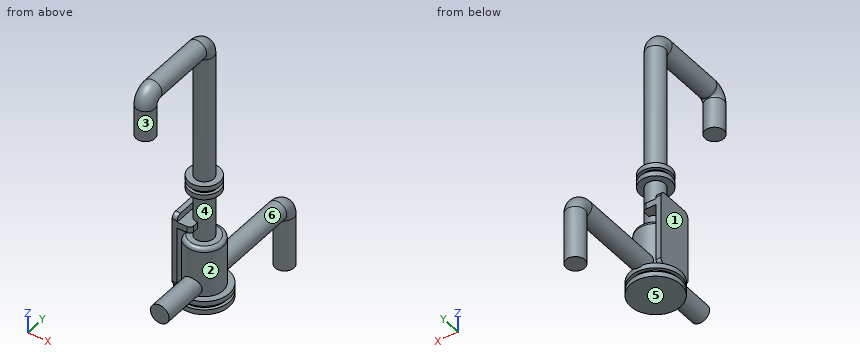
```python
from build123d import *

# Parameters (mm, degrees)
F1_R      = 0.75
F3_R      = 1.5
F3_R_2    = 0.75
F4_DEPTH  = 4
F6_DEPTH  = 6
F7_R      = 0.4
F8_R      = 2
F9_DEPTH  = 0.4
F10_R     = 1.75
F11_DEPTH = 0.3
F12_R     = 2
F12_R_2   = 1.75
F13_DEPTH = 0.4
F14_W     = 3
F14_H     = 0.5
F15_DEPTH = 1.5
F16_R     = 0.3
F18_R     = 1.25
F18_R_2   = 0.75
F19_DEPTH = 0.4
F20_R     = 1
F20_R_2   = 0.75
F21_DEPTH = 0.3
F22_R     = 1.25
F22_R_2   = 1
F22_R_3   = 0.75
F23_DEPTH = 0.4
F24_R     = 0.3
F27_R     = 0.75


with BuildPart() as f2:
    # F2: sweep along a path in F0
    with BuildLine(Plane.YZ) as f2_path:
        Line((0, 0), (0, 2.5))
        ThreePointArc((0, 2.5), (0.2343145751, 3.0656854249), (0.8, 3.3))
        Line((0.8, 3.3), (5.8, 3.3))
        ThreePointArc((5.8, 3.3), (6.3656854249, 3.0656854249), (6.6, 2.5))
        Line((6.6, 2.5), (6.6, -16.7))
    # F1 (on Top) → F2 (sweep)
    with BuildSketch(Plane.XY):
        Circle(F1_R)
    sweep(path=f2_path.line)

    # F3 (on face) → F4 (join)
    with BuildSketch(Plane(origin=(0, 0, -16.7), x_dir=(1, 0, 0), z_dir=(0, 0, -1))):
        with Locations((0, -6.6)):
            Circle(F3_R)
        with Locations((0, -6.6)):
            Circle(F3_R_2, mode=Mode.SUBTRACT)
    extrude(amount=-F4_DEPTH)

    # F5 (on face) → F6 (join)
    with BuildSketch(Plane(origin=(0, 0, -16.7), x_dir=(1, 0, 0), z_dir=(0, 0, -1))):
        with BuildLine():
            ThreePointArc((-1.1, -7.6198039027), (-1.3964240044, -7.1477225575), (-1.5, -6.6))
            Line((-1.5, -6.6), (-1.5, -8.1))
            Line((-1.5, -8.1), (-1.1, -8.1))
            Line((-1.1, -8.1), (-1.1, -7.6198039027))
        make_face()
        with BuildLine():
            Line((-1.5, -5.1), (-1.5, -6.6))
            ThreePointArc((-1.5, -6.6), (-1.3964240044, -6.0522774425), (-1.1, -5.5801960973))
            Line((-1.1, -5.5801960973), (-1.1, -5.1))
            Line((-1.1, -5.1), (-1.5, -5.1))
        make_face()
        with BuildLine():
            ThreePointArc((-1.1, -5.5801960973), (-1.3964240044, -6.0522774425), (-1.5, -6.6))
            ThreePointArc((-1.5, -6.6), (-1.3964240044, -7.1477225575), (-1.1, -7.6198039027))
            Line((-1.1, -7.6198039027), (-1.1, -5.5801960973))
        make_face()
    extrude(amount=-F6_DEPTH)

    # F7
    f7_edges = [f2.edges().sort_by_distance(p)[0] for p in [
        (-1.3, 8.1, -10.7),
        (-1.3, 5.1, -10.7),
        (-1.3, 8.1, -16.7),
        (-1.3, 5.1, -16.7),
    ]]
    fillet(f7_edges, radius=F7_R)

    # F8 (on face) → F9 (join)
    with BuildSketch(Plane(origin=(0, 0, -16.7), x_dir=(1, 0, 0), z_dir=(0, 0, -1))):
        with Locations((0, -6.6)):
            Circle(F8_R)
        with BuildLine():
            Line((-1.1, -5.5), (-1.1, -5.5801960973))
            ThreePointArc((-1.1, -5.5801960973), (1.5, -6.6), (-1.1, -7.6198039027))
            Line((-1.1, -7.6198039027), (-1.1, -7.7))
            Line((-1.1, -7.7), (-1.5, -7.7))
            Line((-1.5, -7.7), (-1.5, -6.6))
            Line((-1.5, -6.6), (-1.5, -5.5))
            Line((-1.5, -5.5), (-1.1, -5.5))
        make_face(mode=Mode.SUBTRACT)
        with BuildLine():
            ThreePointArc((-1.1, -7.6198039027), (1.5, -6.6), (-1.1, -5.5801960973))
            Line((-1.1, -5.5801960973), (-1.1, -5.5))
            Line((-1.1, -5.5), (-1.5, -5.5))
            Line((-1.5, -5.5), (-1.5, -6.6))
            Line((-1.5, -6.6), (-1.5, -7.7))
            Line((-1.5, -7.7), (-1.1, -7.7))
            Line((-1.1, -7.7), (-1.1, -7.6198039027))
        make_face()
    extrude(amount=F9_DEPTH)

    # F10 (on face) → F11 (join)
    with BuildSketch(Plane(origin=(0, 0, -17.1), x_dir=(1, 0, 0), z_dir=(0, 0, -1))):
        with Locations((0, -6.6)):
            Circle(F10_R)
    extrude(amount=F11_DEPTH)

    # F12 (on face) → F13 (join)
    with BuildSketch(Plane(origin=(0, 0, -17.4), x_dir=(1, 0, 0), z_dir=(0, 0, -1))):
        with Locations((0, -6.6)):
            Circle(F12_R)
        with Locations((0, -6.6)):
            Circle(F12_R_2, mode=Mode.SUBTRACT)
        with Locations((0, -6.6)):
            Circle(F12_R_2)
    extrude(amount=F13_DEPTH)

    # F14 (on face) → F15 (join, through all)
    with BuildSketch(Plane(origin=(-1.5, 0, 0), x_dir=(0, -1, 0), z_dir=(-1, 0, 0))):
        with Locations((-6.6, -11.45)):
            Rectangle(F14_W, F14_H)
    extrude(amount=-F15_DEPTH)

    # F16
    f16_edges = [f2.edges().sort_by_distance(p)[0] for p in [
        (0, 8.1, -11.45),
        (0, 5.1, -11.45),
    ]]
    fillet(f16_edges, radius=F16_R)

    # F18 (on offset) → F19 (join)
    with BuildSketch(Plane(origin=(0, 0, -8.8), x_dir=(1, 0, 0), z_dir=(0, 0, -1))):
        with Locations((0, -6.6)):
            Circle(F18_R)
        with Locations((0, -6.6)):
            Circle(F18_R_2, mode=Mode.SUBTRACT)
    extrude(amount=-F19_DEPTH)

    # F20 (on face) → F21 (join)
    with BuildSketch(Plane.XY.offset(-8.4)):
        with Locations((0, 6.6)):
            Circle(F20_R)
        with Locations((0, 6.6)):
            Circle(F20_R_2, mode=Mode.SUBTRACT)
    extrude(amount=F21_DEPTH)

    # F22 (on face) → F23 (join)
    with BuildSketch(Plane.XY.offset(-8.1)):
        with Locations((0, 6.6)):
            Circle(F22_R)
        with Locations((0, 6.6)):
            Circle(F22_R_2, mode=Mode.SUBTRACT)
        with Locations((0, 6.6)):
            Circle(F22_R_2)
        with Locations((0, 6.6)):
            Circle(F22_R_3, mode=Mode.SUBTRACT)
    extrude(amount=F23_DEPTH)

    # F24
    f24_edges = [f2.edges().sort_by_distance(p)[0] for p in [
        (1.5, 6.6, -12.7),
    ]]
    fillet(f24_edges, radius=F24_R)

    # F29: sweep along a path in F28
    with BuildLine(Plane.YZ) as f29_path:
        Line((1.6, -16.0744767636), (6.6, -16.0744767636))
        Line((6.6, -16.0744767636), (14.8, -16.0744767636))
        ThreePointArc((14.8, -16.0744767636), (15.3656854249, -16.3087913387), (15.6, -16.8744767636))
        Line((15.6, -16.8744767636), (15.6, -21.0744767636))
    # F27 (on plane+point) → F29 (sweep)
    with BuildSketch(Plane.XZ.offset(-6.6)):
        with Locations((0, -16.0744767636)):
            Circle(F27_R)
    sweep(path=f29_path.line)


solid = f2.part
```
CAD build for the part. Positions are in the model's coordinates, mm. Face numbers are marked on the shaded views. A direction names the side the tool comes from. Round coordinates to 2 decimals unless told otherwise and drop trailing zeros. Write each loop counter-clockwise with the first axis right and the second up, starting at its lowest first coordinate (ties: lowest second). Pieces come first, ordered by that corner, then holes. Notation, with made-up numbers: (-10.75, 88) - (45.25, 88) arc R24 cw to (45.25, 109) - close; hole circle Ø1 at (83, 76). An arc over 180 degrees is marked (long way). Return JSON: item names as keys, results as strings. Group by question number.
Item 1: 3-axis set-ups, long thin cutter, end or side, ignore diameter. For the marked faces 1, 2 and 3: which of +Z, -Z, +X, -X, +Y, -Y reach the whole face in a straight line?
Item 2: Band-saw the part on A-A on z = -5.5. List the corners of the cut face in (x, y), plus the area to 3 significant figures.
Item 3: Probe probe 1 along Z at (x, y) = (0.6, 2); probe 2 along Z at (x, y) = (1, 8); probe 3 along Z at (x, y) = (-0.65, 4). List the from-to ranges inside material, lowest first.
Item 4: Mould opens along Y. For the marked faces 4, 5 and 6 say: +Y half, -Y half, draft (parallel to the pull), parting line (faces both ways), or undercut.
Item 5: Flat gauge pins, fed straight in: pin 1 Ø1.3 at (x, y) = (1, 6) entering from +Z; pin 2 Ø1.2 at (x, z) = (0, -16) entering from -Y; pin 3 Ø1 at (x, z) = (-1, -12.5) entering from +Y. Where does each tip first touch, or does it go through?
Resolved:
{
 "1": {"face 1": "+Z, -X, +Y, -Y", "face 2": "none", "face 3": "-Z"},
 "2": {"outline": "circle Ø1.5 at (0, 6.6)", "area": "1.77 mm²"},
 "3": {"probe 1": "z = -16.52 to -15.62, 2.85 to 3.75", "probe 2": "z = -17.8 to -16.7", "probe 3": "z = -16.45 to -15.7, 2.93 to 3.67"},
 "4": {"face 4": "parting line", "face 5": "draft", "face 6": "undercut"},
 "5": {"pin 1": "stops at z = 3.96", "pin 2": "stops at y = 1.6", "pin 3": "stops at y = 8.1"}
}
